CAD build for the part. Positions are in the model's coordinates, mm. A direction names the side the tool comes from. Round coordinates to 2 decimals unless told otherwise and drop trailing zeros. Loops run counter-clockwise (first coordinate to the right, second up) from the corner with the lowest first, then second, coordinate; pieces in that order, holes last. Notation, with made-up numbers: (60, 44.5) - (119, 44.5) arc R31 cw to (119, 77.5) - close; hole circle Ø10 at (6, 50.5). An arc over 180 degrees is marked (long way). Use one line per item in the form item = value.
from build123d import *

# Parameters (mm, degrees)
F1_DEPTH = 25.4
F2_W     = 82.763381
F2_H     = 96.530288
F3_DEPTH = 19.05


with BuildPart() as f1:
    # F0 (on Top) → F1 (new body)
    with BuildSketch(Plane.XY):
        Polygon((-13.685921, 33.769403), (-13.523958, 42.191509), (-34.579221, 42.191509), (-34.579221, 33.769403), (-28.100679, 33.769403), (-28.100679, -13.361994), (-34.579221, -13.361994), (-34.579221, -21.460174), (-19.1162, -21.460174), (-21.946063, -33.445477), (-28.424606, -33.445477), (-28.424606, -42.029545), (-7.045416, -42.029545), (-7.045416, -33.445477), (-11.904322, -33.445477), (-8.665049, -21.460174), (5.101852, -21.460174), (8.477995, -33.445477), (1.86258, -33.445477), (1.86258, -42.029545), (23.403736, -42.029545), (23.403736, -34.255296), (17.249119, -34.255296), (14.009847, -21.460174), (25.023371, -21.460174), (25.023371, -4.453998), (16.439302, -4.453998), (16.439302, -13.200031), (12.066286, -13.200031), (3.79868, 20.650355), (-8.665049, 20.650355), (-17.087156, -13.038067), (-19.840537, -13.038067), (-19.840537, 33.769403), align=None)
        Polygon((-7.045416, -12.552176), (-2.510434, 10.770578), (2.510437, -12.552176), align=None, mode=Mode.SUBTRACT)
    extrude(amount=F1_DEPTH)

    # F2 (on Top) → F3 (join)
    with BuildSketch(Plane.XY):
        with Locations((-6.478544, -0.242945)):
            Rectangle(F2_W, F2_H)
    extrude(amount=F3_DEPTH)


solid = f1.part
1) Slice it at C-C (y = -40.5). Write the cut outline in (x, z).
Report:
outline = (-47.86, 0) - (34.9, 0) - (34.9, 19.05) - (23.4, 19.05) - (23.4, 25.4) - (1.86, 25.4) - (1.86, 19.05) - (-7.05, 19.05) - (-7.05, 25.4) - (-28.42, 25.4) - (-28.42, 19.05) - (-47.86, 19.05) - close
2) Drill centre lines: probe 1 along Y at (x, z) = (-25.5, 21.75); probe 2 along Z at (x, y) = (15, -1); probe 3 along X at (y, z) = (30.5, 21). Where is each one in solid material? Low to high.
Report:
probe_1 = -42.03 to -33.45, -21.46 to 42.19
probe_2 = 0 to 19.05
probe_3 = -28.1 to -19.84
3) Two-plate mould, pull along Y, no slides. Class faces 1 (the flat face through (-25, -33.445, 22)), 2 (the flat face through (-34.579, 38, 22)), 3 (the flat face through (-7, 48.022, 9)): +Y half, -Y half, draft (parallel to the pull), parting line (faces both ways), or undercut.
Report:
face_1 = undercut
face_2 = draft
face_3 = +Y half
4) Slice it at A-A (y = -18). Write the cut outline in (x, z).
Report:
outline = (-47.86, 0) - (34.9, 0) - (34.9, 19.05) - (25.02, 19.05) - (25.02, 25.4) - (-34.58, 25.4) - (-34.58, 19.05) - (-47.86, 19.05) - close
5) Flat gauge pins, fed straight in: pin 1 (3 mm diameter, centred on y = -37.5, z = 22, fed in from -X); pin 2 (7 mm diameter, centred on y = -16.5, z = 21, fed in from -X); pin 3 (3 mm diameter, centred on y = 39.5, z = 21, fed in from -X); pin 4 (1.9 mm diameter, centred on x = 4, z = 21, fed in from +Y). Where does each tip first touch, or does it go through?
Report:
pin_1 = -28.42
pin_2 = -47.86
pin_3 = -34.58
pin_4 = 20.65
6) Slice it at D-D (x = 10.5). Write the cut outline in (y, z), plus the area to 3 significant figures.
Report:
outline = (-48.51, 0) - (48.02, 0) - (48.02, 19.05) - (-6.79, 19.05) - (-6.79, 25.4) - (-42.03, 25.4) - (-42.03, 19.05) - (-48.51, 19.05) - close
area = 2,060 mm^2
7) Slice it at B-B (x = 21.5). Write the cut outline in (y, z), plus the area to 3 significant figures.
Report:
outline = (-48.51, 0) - (48.02, 0) - (48.02, 19.05) - (-4.45, 19.05) - (-4.45, 25.4) - (-21.46, 25.4) - (-21.46, 19.05) - (-34.26, 19.05) - (-34.26, 25.4) - (-42.03, 25.4) - (-42.03, 19.05) - (-48.51, 19.05) - close
area = 2,000 mm^2
8) Tool access for faces 4 (the flat face through (21, -4.454, 22)), 5 (the flat face through (-12.817, 4.042, 22.181)), 6 (the flat face through (-28.425, -38, 22)): list every direction of +Z, -Z, +X, -X, +Y, -Y with a clear straight run to the whole face (end or side of a thin tool).
Report:
face_4 = +Z, +X, +Y
face_5 = +Z
face_6 = +Z, -X, -Y
